Geometry check sheet. Reference: the model listing, model coordinates, mm. A direction names the side the tool comes from. Round coordinates to 2 decimals unless told otherwise and drop trailing zeros. Loops run counter-clockwise (first coordinate to the right, second up) from the corner with the lowest first, then second, coordinate; pieces in that order, holes last. Notation, with made-up numbers: (-39, 84.5) -> (-34, 84.5) arc R24 ccw to (-34, 117.5) -> close; hole circle Ø6 at (-27.75, 7.5). An arc over 180 degrees is marked (long way). Use a Markdown table: item, result. Add a question column.
Q1. Set-up check for faces 1 (the face through (10, 0, -1)), 2 (the face through (-0.06, 2.03, -7.01)), 3 (the face through (-1, 4, -2)), 4 (the face through (17, 6, 0)), 5 (the face through (24.1, 2.03, 3.14)): record each of +Z, -Z, +X, -X, +Y, -Y from which the full face is reachable in a straight line by a thin tool's end or side.
Q2. Sectioned sample at C-C, the plane x = 0. Enter the section's corners in (y, z), then the cut area to 3 significant figures.
Q3. Sectioned sample at D-D, the plane z = 0. Enter the section's corners in (x, y).
Q4. Sectioned sample at A-A, the plane z = -4.75. Enter the section's corners in (x, y), then the cut area to 3 significant figures.
Q5. Material ranges on L1, parallel to X at y = 2, z = 0; L2, parallel to Z at x = 10.5, y = 10; L3, parallel to Y at x = 21.75, z = -5, recorded low to high.
Q6. Release check for a two-part mould opening along Z. For faces 6 (the face through (21.686, 1.972, -0.221)), 7 (the face through (-3, 2, -8)), 8 (the face through (3, 6, 0)), 9 (the face through (-1.66, 1.97, -0.37)) record: released by +Z, released by -Z, zero draft, split by the parting line, or undercut.
Q7. Sectioned sample at B-B, the plane y = 2.75. Enter the section's corners in (x, z), then the cut area to 3 significant figures.
Q8. Gauge pin test, flat ends, axial feed: P1, Ø4, axis at x = 20, z = 0, coming from the +Y side; P2, Ø1.5, axis at x = 5.5, y = 8.5, coming from the -Z side; P3, Ø3, axis at y = 10, z = -3.5, coming from the +X side; P4, Ø3, axis at x = 0, z = 0, coming from the +Y side. Record the tip position at first contact, or that the pin passes through.
```python
from build123d import *

# Parameters (mm, degrees)
SKETCH1_W           = 30
SKETCH1_H           = 8
SKETCH1_R           = 1.7
BOSS_EXTRUDE1_DEPTH = 4
FILLET1_R           = 3
SKETCH2_W           = 5.95
SKETCH2_H           = 4
BOSS_EXTRUDE2_DEPTH = 4
SKETCH3_W           = 14
SKETCH3_H           = 8
BOSS_EXTRUDE3_DEPTH = 8
CHAMFER1_SIZE       = 4
CHAMFER2_SIZE       = 2


with BuildPart() as part:
    # Sketch1 → Boss-Extrude1 (new body)
    with BuildSketch(Plane(origin=(0, 0, 0), x_dir=(1, 0, 0), z_dir=(0, 1, 0))):
        with Locations((10, 0)):
            Rectangle(SKETCH1_W, SKETCH1_H)
        with Locations(Location((0, 0, 0), (0, 0, 270))):
            Circle(SKETCH1_R, mode=Mode.SUBTRACT)
        with Locations(Location((20, 0, 0), (0, 0, 270))):
            Circle(SKETCH1_R, mode=Mode.SUBTRACT)
    extrude(amount=BOSS_EXTRUDE1_DEPTH)

    # Fillet1
    fillet1_edges = [part.edges().sort_by_distance(p)[0] for p in [
        (25, 2, 4),
        (-5, 2, 4),
    ]]
    fillet(fillet1_edges, radius=FILLET1_R)

    # Sketch2 → Boss-Extrude2 (add)
    with BuildSketch(Plane(origin=(0, 4, 0), x_dir=(1, 0, 0), z_dir=(0, 1, 0))):
        with Locations((-2.025, 6)):
            Rectangle(SKETCH2_W, SKETCH2_H)
        with Locations((22.025, 6)):
            Rectangle(SKETCH2_W, SKETCH2_H)
    extrude(amount=-BOSS_EXTRUDE2_DEPTH)

    # Sketch3 → Boss-Extrude3 (add)
    with BuildSketch(Plane(origin=(0, 4, 0), x_dir=(1, 0, 0), z_dir=(0, 1, 0))):
        with Locations((10, 0)):
            Rectangle(SKETCH3_W, SKETCH3_H)
    extrude(amount=BOSS_EXTRUDE3_DEPTH)

    # Chamfer1
    chamfer1_edges = [part.edges().sort_by_distance(p)[0] for p in [
        (17, 12, 0),
        (3, 12, 0),
    ]]
    chamfer(chamfer1_edges, length=CHAMFER1_SIZE)

    # Chamfer2
    chamfer2_edges = [part.edges().sort_by_distance(p)[0] for p in [
        (0.95, 2, -8),
        (19.05, 2, -8),
    ]]
    chamfer(chamfer2_edges, length=CHAMFER2_SIZE)


solid = part.part
```
Values:
| question | item | result |
|---|---|---|
| 1 | face 1 | +Z, -Z, +X, -X, -Y |
| 1 | face 2 | -Z, +Y, -Y |
| 1 | face 3 | +Z, -Z, -X, +Y |
| 1 | face 4 | +Z, -Z, +X, +Y |
| 1 | face 5 | +Z, +X, +Y, -Y |
| 2 | outline | (0, -6.95) -> (4, -6.95) -> (4, -1.7) -> (0, -1.7) -> close; (0, 1.7) -> (4, 1.7) -> (4, 4) -> (0, 4) -> close |
| 2 | area | 30.2 mm^2 |
| 3 | outline | (-5, 0) -> (-1.7, 0) -> (-1.7, 4) -> (-5, 4) -> close; (1.7, 0) -> (18.3, 0) -> (18.3, 4) -> (17, 4) -> (17, 8) -> (13, 12) -> (7, 12) -> (3, 8) -> (3, 4) -> (1.7, 4) -> close; (21.7, 0) -> (25, 0) -> (25, 4) -> (21.7, 4) -> close |
| 4 | outline | (-5, 0) -> (0.95, 0) -> (0.95, 4) -> (-5, 4) -> close; (19.05, 0) -> (25, 0) -> (25, 4) -> (19.05, 4) -> close |
| 4 | area | 47.6 mm^2 |
| 5 | L1 | -5 to -1.7, 1.7 to 18.3, 21.7 to 25 |
| 5 | L2 | -4 to 4 |
| 5 | L3 | 0 to 4 |
| 6 | face 6 | undercut |
| 6 | face 7 | released by -Z |
| 6 | face 8 | zero draft |
| 6 | face 9 | undercut |
| 7 | outline | (-5, -8) -> (-1.05, -8) -> (0.95, -6) -> (0.95, -4) -> (19.05, -4) -> (19.05, -6) -> (21.05, -8) -> (25, -8) -> (25, 1) arc R3 ccw to (22, 4) -> (-2, 4) arc R3 ccw to (-5, 1) -> close; hole circle Ø3.4 at (0, 0); hole circle Ø3.4 at (20, 0) |
| 7 | area | 262 mm^2 |
| 8 | P1 | y = 4 |
| 8 | P2 | z = -4 |
| 8 | P3 | x = 16.5 |
| 8 | P4 | through |
